Work out the finished part from the listing and answer in its coordinate system (mm). Give positions to 0.01 mm unless a question says otherwise; leave off trailing zeros. Loops run counter-clockwise (first coordinate to the right, second up) from the corner with the lowest first, then second, coordinate; pieces in that order, holes last. Notation, with made-up numbers: M -3.5,-13.75 L 42.5,-13.75 A26 ccw 42.5,2.25 Z; hole C 39,51 d7. An arc over 180 degrees is marked long. Answer as a JSON object with one key per item and string values. Group by question number.
Autodesk Inventor part; units mm, degrees
ref_plane "YZ Plane" through (0, 0, 0) normal (1, 0, 0) x (0, 1, 0)
ref_plane "XZ Plane" through (0, 0, 0) normal (0, 1, 0) x (-1, 0, 0)
ref_plane "XY Plane" through (0, 0, 0) normal (0, 0, 1) x (1, 0, 0)
sketch "Sketch1" plane through (0, 0, 0) normal (0, 1, 0) x (-1, 0, 0)
  circle A0 centre (0, 0) radius 2.1844
  circle A1 centre (30.353, 0) radius 2.1844
  line L0 (0, -12.7) -> (0, 0)
  circle A2 centre (30.353, -12.7) radius 2.1844
  circle A3 centre (0, -12.7) radius 2.1844
  circle A4 centre (0, -12.7) radius 6.35
  circle A5 centre (0, 0) radius 6.35
  line L1 (30.353, -19.05) -> (0, -19.05)
  line L2 (-6.35, -12.7) -> (-6.35, 0)
  line L3 (0, 6.35) -> (30.353, 6.35)
  line L4 (30.353, 0) -> (31.9405, 0)
  circle A6 centre (31.9405, 0) radius 6.35
  circle A7 centre (31.9405, -12.7) radius 6.35
  line L5 (30.353, 6.35) -> (31.9405, 6.35)
  line L6 (30.353, -19.05) -> (31.9405, -19.05)
  line L7 (38.2905, -12.7) -> (38.2905, 0)
  dimension "d0" = 4.3688
  dimension "d2" = 4.3688
  dimension "d4" = 4.3688
  dimension "d5" = 4.3688
  dimension "d8" = 12.7
  dimension "d9" = 12.7
  dimension "d10" = 1.5875
  dimension "d12" = 12.7
  dimension "d13" = 12.7
extrude "Extrusion1" add sketch "Sketch1" along normal blind 1.5875
properties part number "lbgrippermountpoly"
Item 1: Find the intervals of material crossed by probe 1 along Z at (x, y) = (0, 0.7); probe 2 along Z at (x, y) = (1, 0.25); probe 3 along X at (y, z) = (1.1, 1), in increasing order. Write a range as [from, to].
Item 2: A cutting plane is placed at A-A (y = 0.5). Determine the outline of the cut face in (x, z), and give its area (3 significant figures).
Item 3: Given pin 1 Ø4 at (x, z) = (0, -12.7) entering from +Y, flat-ended and moving along its own axis, determine where the tip first touches the part or whether it passes through.
Item 4: A cutting plane is placed at B-B (x = 1). Determine the outline of the cut face in (y, z).
Item 5: For a pull along X with two mould halves and no side action, classify faces 1 (the cylindrical face through (-29.879, 0.783, -10.568)), 2 (the cylindrical face through (-36.38, 0.78, 4.54)), 3 (the flat face through (6.35, 1, -6)) as pulls with the +X half, pulls with the -X half, needs draft (parallel to the pull), parting line crosses it, or undercut.
Item 6: A cutting plane is placed at C-C (z = -0.5). Determine the outline of the cut face in (x, y).
The answers:
{
 "1": {"probe 1": "z = [-19.05, -14.88], [-10.52, -2.18], [2.18, 6.35]", "probe 2": "z = [-18.97, -14.64], [-10.76, -1.94], [1.94, 6.27]", "probe 3": "x = [-38.21, -32.3], [-28.41, -1.94], [1.94, 6.27]"},
 "2": {"outline": "M -38.29,-12.7 A6.35 ccw -31.94,-19.05 L 0,-19.05 A6.35 ccw 6.35,-12.7 L 6.35,0 A6.35 ccw 0,6.35 L -31.94,6.35 A6.35 ccw -38.29,0 Z; hole C -30.35,-12.7 d4.37; hole C -30.35,0 d4.37; hole C 0,-12.7 d4.37; hole C 0,0 d4.37", "area": "1,040 mm^2"},
 "3": {"pin 1": "passes through"},
 "4": {"outline": "M 0,-18.97 L 1.59,-18.97 L 1.59,-14.64 L 0,-14.64 Z; M 0,-10.76 L 1.59,-10.76 L 1.59,-1.94 L 0,-1.94 Z; M 0,1.94 L 1.59,1.94 L 1.59,6.27 L 0,6.27 Z"},
 "5": {"face 1": "undercut", "face 2": "pulls with the -X half", "face 3": "pulls with the +X half"},
 "6": {"outline": "M -38.29,0 L -32.48,0 L -32.48,1.59 L -38.29,1.59 Z; M -28.23,0 L -2.13,0 L -2.13,1.59 L -28.23,1.59 Z; M 2.13,0 L 6.35,0 L 6.35,1.59 L 2.13,1.59 Z"}
}
